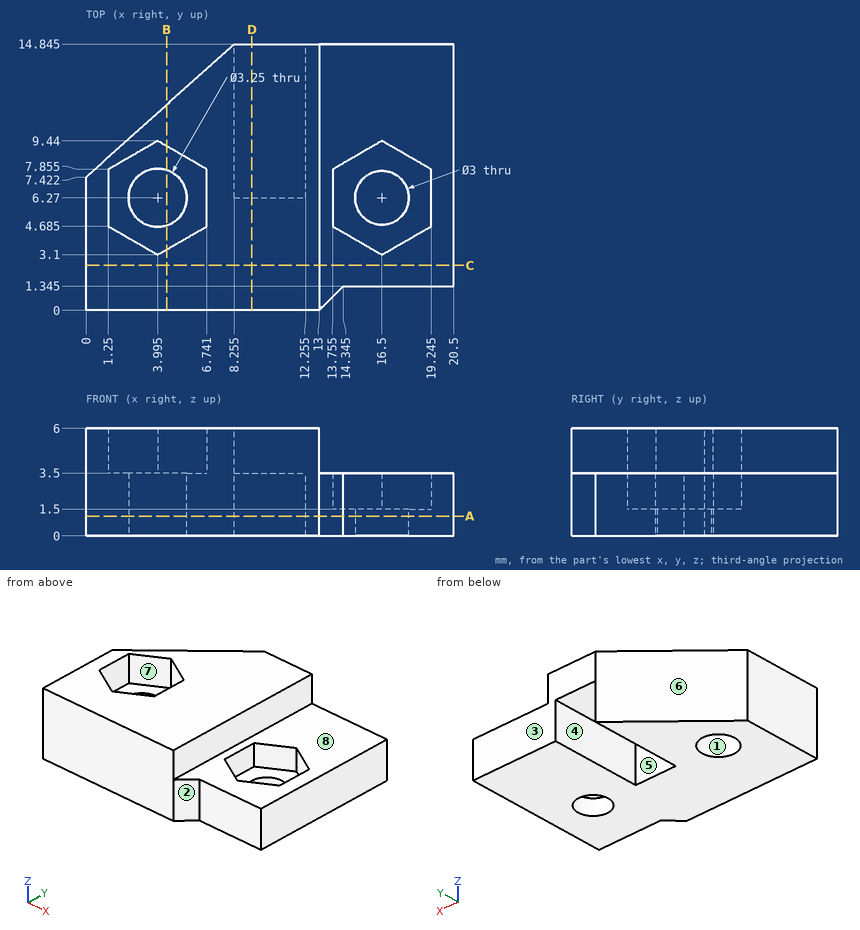
Study the drawing (mm; zero at the part's minimum x, y, z) and answer. A direction names the side the tool comes from. Give positions to 0.01 mm unless a question says otherwise; leave off trailing zeros. Order: outer loops, then holes, each group sorted by start corner. A loop starts at its lowest first (then second) coordinate and runs counter-clockwise, first axis right, second up. Notation, with made-up numbers: (56.25, -40) - (70.25, -40) arc R27 cw to (70.25, -23) - close; hole circle Ø8 at (55.25, 61). An arc over 180 degrees is marked (long way). Answer in a Markdown table with one row per item. Add a question column.
Q1. The part is cut by section C-C (y = 2.5). Determine the outline of the cut face in (x, z), then the cut area to 3 significant figures.
Q2. The part is cut by section A-A (z = 1.1). Give the number of separate pieces and of enclosed holes in the cut face, then the cut area to 3 significant figures.
Q3. For a pull along Y with two mould halves and no side action, classify the marked faces 1, 2, 3 and 4 as released by +Y, released by -Y, zero draft, split by the parting line, or undercut.
Q4. Find the intervals of material crossed by line 1 along Y through (x, z) = (16.5, 1.1) (1 decimal); line 2 along X through (y, z) = (7.5, 0.95) (1 decimal); line 3 along Z through (x, y) = (9.5, 7.5), in increasing order. Write a range as [from, to].
Q5. Given P1, Ø3.5, axis at x = 16.5, y = 6.27, coming from the +Z side; P2, Ø1.5, axis at x = 18, y = 8.5, coming from the +Z side; P3, Ø2, axis at y = 8, z = 5, coming from the +X side, each flat-ended and moving along its own axis, determine where each tip first touches the part or whether it passes through.
Q6. The part is cut by section D-D (x = 9.25). Determine the outline of the cut face in (y, z) (1 decimal).
Q7. Which of the six approach directions +Z, -Z, +X, -X, +Y, -Y give full straight-line access (tool end or side, diameter ignored) to the marked faces 5, 6, 7 and 8?
Q8. The part is cut by section B-B (x = 4.5). Determine the outline of the cut face in (y, z) (1 decimal), then the cut area to 3 significant figures.
Determined:
| question | item | result |
|---|---|---|
| 1 | outline | (0, 0) - (20.5, 0) - (20.5, 3.5) - (13, 3.5) - (13, 6) - (0, 6) - close |
| 1 | area | 104 mm² |
| 2 | separate pieces | 1 |
| 2 | enclosed holes | 2 |
| 2 | area | 215 mm² |
| 3 | face 1 | undercut |
| 3 | face 2 | released by -Y |
| 3 | face 3 | released by +Y |
| 3 | face 4 | zero draft |
| 4 | line 1 | y = [1.3, 4.8], [7.8, 14.8] |
| 4 | line 2 | x = [0.1, 2.9], [5.1, 8.3], [12.3, 15.6], [17.4, 20.5] |
| 4 | line 3 | z = [3.5, 6] |
| 5 | P1 | stops at z = 1.5 |
| 5 | P2 | stops at z = 3.5 |
| 5 | P3 | stops at x = 13 |
| 6 | outline | (0, 0) - (6.3, 0) - (6.3, 3.5) - (14.8, 3.5) - (14.8, 6) - (0, 6) - close |
| 7 | face 5 | -Z, +Y |
| 7 | face 6 | +Z, -Z, -X, +Y |
| 7 | face 7 | +Z |
| 7 | face 8 | +Z, +X, +Y, -Y |
| 8 | outline | (0, 0) - (4.7, 0) - (4.7, 3.5) - (3.4, 3.5) - (3.4, 6) - (0, 6) - close; (7.8, 0) - (11.5, 0) - (11.5, 6) - (9.1, 6) - (9.1, 3.5) - (7.8, 3.5) - close |
| 8 | area | 43.6 mm² |
